from build123d import *

# Parameters (mm, degrees)
SKETCH1_W                = 75.15
SKETCH1_H                = 75.15
SKETCH1_W_2              = 14
SKETCH1_H_2              = 14
BOSS_EXTRUDE1_DEPTH      = 3
SKETCH2_R                = 1
CUT_EXTRUDE1_DEPTH       = 3
CHAMFER1_SIZE            = 1
CHAMFER1_OF_MIRROR1_SIZE = 1
MOVE_FACE1_BY            = 0.2
MOVE_FACE1_2_BY          = 0.2
MOVE_FACE1_3_BY          = 0.2
MOVE_FACE1_4_BY          = 0.2


with BuildPart() as part:
    # Sketch1 → Boss-Extrude1 (new body)
    with BuildSketch(Plane(origin=(0, 0, 0), x_dir=(1, 0, 0), z_dir=(0, 1, 0))):
        Rectangle(SKETCH1_W, SKETCH1_H)
        with Locations((-9.525, 28.575)):
            Rectangle(SKETCH1_W_2, SKETCH1_H_2, mode=Mode.SUBTRACT)
        with Locations((-28.575, 28.575)):
            Rectangle(SKETCH1_W_2, SKETCH1_H_2, mode=Mode.SUBTRACT)
        with Locations((9.525, 28.575)):
            Rectangle(SKETCH1_W_2, SKETCH1_H_2, mode=Mode.SUBTRACT)
        with Locations((28.575, 28.575)):
            Rectangle(SKETCH1_W_2, SKETCH1_H_2, mode=Mode.SUBTRACT)
        with Locations((-9.525, 9.525)):
            Rectangle(SKETCH1_W_2, SKETCH1_H_2, mode=Mode.SUBTRACT)
        with Locations((9.525, 9.525)):
            Rectangle(SKETCH1_W_2, SKETCH1_H_2, mode=Mode.SUBTRACT)
        with Locations((28.575, 9.525)):
            Rectangle(SKETCH1_W_2, SKETCH1_H_2, mode=Mode.SUBTRACT)
        with Locations((-9.525, -9.525)):
            Rectangle(SKETCH1_W_2, SKETCH1_H_2, mode=Mode.SUBTRACT)
        with Locations((9.525, -9.525)):
            Rectangle(SKETCH1_W_2, SKETCH1_H_2, mode=Mode.SUBTRACT)
        with Locations((28.575, -9.525)):
            Rectangle(SKETCH1_W_2, SKETCH1_H_2, mode=Mode.SUBTRACT)
        with Locations((-9.525, -28.575)):
            Rectangle(SKETCH1_W_2, SKETCH1_H_2, mode=Mode.SUBTRACT)
        with Locations((9.525, -28.575)):
            Rectangle(SKETCH1_W_2, SKETCH1_H_2, mode=Mode.SUBTRACT)
        with Locations((28.575, -28.575)):
            Rectangle(SKETCH1_W_2, SKETCH1_H_2, mode=Mode.SUBTRACT)
        with Locations((-28.575, 9.525)):
            Rectangle(SKETCH1_W_2, SKETCH1_H_2, mode=Mode.SUBTRACT)
        with Locations((-28.575, -9.525)):
            Rectangle(SKETCH1_W_2, SKETCH1_H_2, mode=Mode.SUBTRACT)
        with Locations((-28.575, -28.575)):
            Rectangle(SKETCH1_W_2, SKETCH1_H_2, mode=Mode.SUBTRACT)
    extrude(amount=BOSS_EXTRUDE1_DEPTH)

    # Sketch2 → Cut-Extrude1 (cut)
    with BuildSketch(Plane(origin=(0, 3, 0), x_dir=(1, 0, 0), z_dir=(0, 1, 0))):
        with Locations(Location((-19.05, 19.05, 0), (0, 0, 270))):
            Circle(SKETCH2_R)
        with Locations(Location((-28.575, -19.05, 0), (0, 0, 270))):
            Circle(SKETCH2_R)
    cut_extrude1 = extrude(amount=-CUT_EXTRUDE1_DEPTH, mode=Mode.SUBTRACT)

    # Chamfer1
    chamfer1_edges = [part.edges().sort_by_distance(p)[0] for p in [
        (-19.05, 3, -20.05),
        (-28.575, 3, 18.05),
    ]]
    chamfer(chamfer1_edges, length=CHAMFER1_SIZE)

    # Mirror1: Cut-Extrude1 across plane
    add(cut_extrude1.mirror(Plane(origin=(0, 0, 0), x_dir=(0, 0, 1), z_dir=(1, 0, 0))), mode=Mode.SUBTRACT)

    # Chamfer1 of Mirror1
    chamfer1_of_mirror1_edges = [part.edges().sort_by_distance(p)[0] for p in [
        (19.05, 3, -20.05),
        (28.575, 3, 18.05),
    ]]
    chamfer(chamfer1_of_mirror1_edges, length=CHAMFER1_OF_MIRROR1_SIZE)

    # Move Face1: a face moved inward by 0.2
    extrude(part.faces().sort_by_distance((37.575, 1.5, 0))[0], amount=MOVE_FACE1_BY, dir=(-1, 0, 0), mode=Mode.SUBTRACT)

    # Move Face1 2: a face moved inward by 0.2
    extrude(part.faces().sort_by_distance((0, 1.5, -37.575))[0], amount=MOVE_FACE1_2_BY, dir=(0, 0, 1), mode=Mode.SUBTRACT)

    # Move Face1 3: a face moved inward by 0.2
    extrude(part.faces().sort_by_distance((0, 1.5, 37.575))[0], amount=MOVE_FACE1_3_BY, dir=(0, 0, -1), mode=Mode.SUBTRACT)

    # Move Face1 4: a face moved inward by 0.2
    extrude(part.faces().sort_by_distance((-37.575, 1.5, 0))[0], amount=MOVE_FACE1_4_BY, dir=(1, 0, 0), mode=Mode.SUBTRACT)


solid = part.part
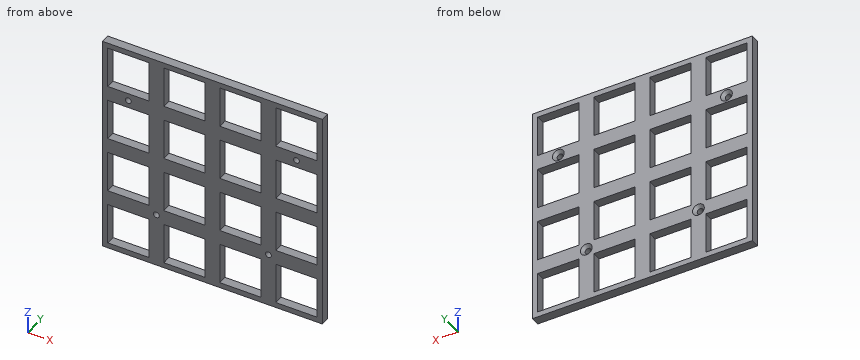
The listing builds one solid part. Answer for the finished solid, in the listing's coordinates (mm). Round coordinates to 2 decimals unless told otherwise and drop trailing zeros. Order: outer loops, then holes, each group sorted by start corner. A loop starts at its lowest first (then second) coordinate and runs counter-clockwise, first axis right, second up. Notation, with made-up numbers: M 18,37.25 L 30,37.25 A31 ccw 30,62.25 Z; hole C -7.75,83 d5. An arc over 180 degrees is marked long. Answer in a Markdown table with one row per item. Add a question column.
1) The part is cut by section A-A on z = 19.05. Determine the outline of the cut face in (x, y) (3 decimals).
2) The part is cut by section D-D on x = -19.05. Determine the outline of the cut face in (y, z) (3 decimals), plus the area to 3 significant figures.
3) Consider line 1 along X through (y, z) = (2.25, -14) (3 decimals); line 2 along X through (y, z) = (0.7, 19.05) (3 decimals). Determine where each line is inside the solid, lowest interval first. Write a range as from..to.
4) The part is cut by section C-C on z = -7.5. Determine the outline of the cut face in (x, y) (3 decimals).
5) The part is cut by section B-B on x = -4. Determine the outline of the cut face in (y, z) (3 decimals), plus the area to 4 significant figures.
Findings below:
| question | item | result |
|---|---|---|
| 1 | outline | M -37.375,0 L -29.575,0 L -29.575,2 L -30.575,3 L -37.375,3 Z; M -27.575,0 L 27.575,0 L 27.575,2 L 26.575,3 L -26.575,3 L -27.575,2 Z; M 29.575,0 L 37.375,0 L 37.375,3 L 30.575,3 L 29.575,2 Z |
| 2 | outline | M 0,-37.375 L 3,-37.375 L 3,-21.05 L 2,-20.05 L 0,-20.05 Z; M 0,-18.05 L 2,-18.05 L 3,-17.05 L 3,37.375 L 0,37.375 Z |
| 2 | area | 217 mm² |
| 3 | line 1 | x = -37.375..-35.575, -21.575..-16.525, -2.525..2.525, 16.525..21.575, 35.575..37.375 |
| 3 | line 2 | x = -37.375..-29.575, -27.575..27.575, 29.575..37.375 |
| 4 | outline | M -37.375,0 L -35.575,0 L -35.575,3 L -37.375,3 Z; M -21.575,0 L -16.525,0 L -16.525,3 L -21.575,3 Z; M -2.525,0 L 2.525,0 L 2.525,3 L -2.525,3 Z; M 16.525,0 L 21.575,0 L 21.575,3 L 16.525,3 Z; M 35.575,0 L 37.375,0 L 37.375,3 L 35.575,3 Z |
| 5 | outline | M 0,-37.375 L 3,-37.375 L 3,-35.575 L 0,-35.575 Z; M 0,-21.575 L 3,-21.575 L 3,-16.525 L 0,-16.525 Z; M 0,-2.525 L 3,-2.525 L 3,2.525 L 0,2.525 Z; M 0,16.525 L 3,16.525 L 3,21.575 L 0,21.575 Z; M 0,35.575 L 3,35.575 L 3,37.375 L 0,37.375 Z |
| 5 | area | 56.25 mm² |
